```python
from build123d import *

# Parameters (mm, degrees)
F0_R     = 6.35
F1_DEPTH = 10.16


# Not quite as in the source:
# - a feature names something its author has since deleted; it is built from what else it names


with BuildPart() as f1:
    # F0 (on Front) → F1 (new body)
    with BuildSketch(Plane.XZ):
        Polygon((-4.8744329511, 71.2045607365), (-75.0909721843, 1.3295207142), (-72.5509721843, 1.3295207142), (-108.4719966685, -34.5915037701), (-103.3919966685, -34.5915037701), (-67.4709721843, 1.3295207142), (-64.9309721843, 1.3295207142), (-20.1762745117, 45.8665532311), (-4.9362745117, 45.8665532311), (5.2855670489, 45.8665532311), (20.3403427678, 45.8665532311), (64.660768747, 1.3295207142), (67.200768747, 1.3295207142), (103.0377074058, -34.6753932222), (108.1177074058, -34.6753932222), (72.2719103919, 1.3207015165), (74.820768747, 1.3295207142), (5.2855670489, 71.2045607365), align=None)
        with Locations((0, 58.6755184585)):
            Circle(F0_R, mode=Mode.SUBTRACT)
    extrude(amount=F1_DEPTH)


solid = f1.part
```
Read the model definition and answer for the solid it produces. Units are mm, in the model's axes. A direction names the side the tool comes from. Coordinates: 2 decimals unless noted, no trailing zeros. Write each loop counter-clockwise with the first axis right and the second up, starting at its lowest first coordinate (ties: lowest second). Pieces come first, ordered by that corner, then holes. Notation, with made-up numbers: (-20, 31.25) -> (4, 31.25) arc R27 ccw to (4, 63.25) -> close; hole circle Ø10 at (-15.5, 39). An arc over 180 degrees is marked (long way). Answer as a JSON object with one key per item and string values.
Q1. A tool of negligible diameter and unlimited length cuts with its end or side. For faces 1 (the flat face through (-1, 0, 50)), 2 (the flat face through (42.2, -5, 23.9)), from which of +Z, -Z, +X, -X, +Y, -Y can it reach the whole face along a straight path? Write none if from no direction.
The answers:
{"face 1": "+Z, -Z, +X, -X, +Y", "face 2": "-Z, +Y, -Y"}
Q2. The part is cut by section D-D on x = 82. Give the vertices of the cut face in (y, z), then the cut area to 3 significant figures.
The answers:
{"outline": "(-10.16, -13.54) -> (0, -13.54) -> (0, -8.45) -> (-10.16, -8.45) -> close", "area": "51.7 mm2"}
Q3. The part is cut by section B-B on z = -4. Give the vertices of the cut face in (x, y).
The answers:
{"outline": "(-77.88, -10.16) -> (-72.8, -10.16) -> (-72.8, 0) -> (-77.88, 0) -> close; (72.51, -10.16) -> (77.57, -10.16) -> (77.57, 0) -> (72.51, 0) -> close"}
Q4. Determine the mould class of faces 3 (the flat face through (-106, -5, -34.592)), 4 (the flat face through (-39.49, -5.01, 36.76)), 5 (the cylindrical face through (-0.83, -5.01, 64.97)), 6 (the flat face through (0, -5, 45.867)) for opening direction X: pulls with the +X half, pulls with the -X half, needs draft (parallel to the pull), parting line crosses it, or undercut.
The answers:
{"face 3": "needs draft", "face 4": "pulls with the -X half", "face 5": "undercut", "face 6": "undercut"}
Q5. The part is cut by section C-C on y = -3. Give the vertices of the cut face in (x, z).
The answers:
{"outline": "(-108.47, -34.59) -> (-103.39, -34.59) -> (-67.47, 1.33) -> (-64.93, 1.33) -> (-20.18, 45.87) -> (20.34, 45.87) -> (64.66, 1.33) -> (67.2, 1.33) -> (103.04, -34.68) -> (108.12, -34.68) -> (72.27, 1.32) -> (74.82, 1.33) -> (5.29, 71.2) -> (-4.87, 71.2) -> (-75.09, 1.33) -> (-72.55, 1.33) -> close; hole circle Ø12.7 at (0, 58.68)"}
Q6. Consider line 1 (Z direction, x = 0, y = -5.5); line 2 (X direction, y = -6.5, z = 64); line 3 (X direction, y = -6.25, z = 39). Determine where each line is inside the solid, lowest interval first. Write a range as [from, to].
The answers:
{"line 1": "z = [45.87, 52.33], [65.03, 71.2]", "line 2": "x = [-12.11, -3.46], [3.46, 12.46]", "line 3": "x = [-37.24, -27.08], [27.17, 37.33]"}
Q7. The part is cut by section A-A on x = 0. Give the vertices of the cut face in (y, z), then the cut area to 3 significant figures.
The answers:
{"outline": "(-10.16, 45.87) -> (0, 45.87) -> (0, 52.33) -> (-10.16, 52.33) -> close; (-10.16, 65.03) -> (0, 65.03) -> (0, 71.2) -> (-10.16, 71.2) -> close", "area": "128 mm2"}
Q8. Flat-ended cylindrical pins translate along their axes: pin 1 Ø0.8 at (x, y) = (66, -5.5) entering from -Z; pin 2 Ø1.5 at (x, z) = (75.5, 2) entering from -Y; pin 3 Ø5 at (x, y) = (-71, -5) entering from +Z; pin 4 Ø1 at (y, z) = (-2.5, 39.5) entering from -X. Find the tip coordinate at first contact, or state that the pin passes through.
The answers:
{"pin 1": "stops at z = 1.33", "pin 2": "passes through", "pin 3": "stops at z = 7.89", "pin 4": "stops at x = -37.24"}
